Could you check a few things on this model? Use its own coordinates, in mm. Face numbers are marked on the shaded views. A direction names the side the tool comes from. Give positions to 0.01 mm unless a question says otherwise; leave off trailing zeros. Loops run counter-clockwise (first coordinate to the right, second up) from the corner with the lowest first, then second, coordinate; pieces in that order, holes last. Notation, with made-up numbers: (20.5, 55.25) - (24.5, 55.25) arc R10 cw to (24.5, 59.25) - close; hole circle Ø5 at (45.25, 34.25). An arc over 180 degrees is marked (long way). Answer in a Markdown table with one row per item. Add a question column.
```python
from build123d import *

# Parameters (mm, degrees)
SKETCH_1_W      = 3
SKETCH_1_H      = 17
EXTRUDE_1_DEPTH = 2.5
SKETCH_1_3_W    = 3
SKETCH_1_3_H    = 17
EXTRUDE_2_DEPTH = 2.5
FILLET_1_R      = 2


with BuildPart() as part:
    # Sketch 1 → Extrude 1 (new body)
    with BuildSketch(Plane(origin=(0, 0, 0), x_dir=(1, 0, 0), z_dir=(0, 1, 0))):
        Polygon((0, 15), (0, 17), (-15, 17), (-25, 6.390453713), (-25, 0), (0, 0), (0, 2), (-24.2, 2), (-24.2, 5), (0, 5), (0, 7), (-19.2, 7), (-19.2, 10), (0, 10), (0, 12), (-12.2, 12), (-12.2, 15), align=None)
        Polygon((5.5, 17), (0, 17), (0, 15), (-12.2, 15), (-12.2, 12), (0, 12), (0, 10), (-19.2, 10), (-19.2, 7), (0, 7), (0, 5), (-24.2, 5), (-24.2, 2), (0, 2), (0, 0), (5.5, 0), align=None)
        with Locations((7, 8.5)):
            Rectangle(SKETCH_1_W, SKETCH_1_H)
    extrude(amount=-EXTRUDE_1_DEPTH)

    # Sketch 1_3 → Extrude 2 (add)
    with BuildSketch(Plane(origin=(0, 0, 0), x_dir=(1, 0, 0), z_dir=(0, 1, 0))):
        Polygon((0, 15), (0, 17), (-15, 17), (-25, 6.390453713), (-25, 0), (0, 0), (0, 2), (-24.2, 2), (-24.2, 5), (0, 5), (0, 7), (-19.2, 7), (-19.2, 10), (0, 10), (0, 12), (-12.2, 12), (-12.2, 15), align=None)
        with Locations((7, 8.5)):
            Rectangle(SKETCH_1_3_W, SKETCH_1_3_H)
    extrude(amount=EXTRUDE_2_DEPTH)

    # Fillet 1
    fillet_1_edges = [part.edges().sort_by_distance(p)[0] for p in [
        (8.5, 0, -17),
        (8.5, 0, 0),
        (-25, 0, 0),
        (-25, 0, -6.390453713),
        (-15, 0, -17),
    ]]
    fillet(fillet_1_edges, radius=FILLET_1_R)


solid = part.part
```
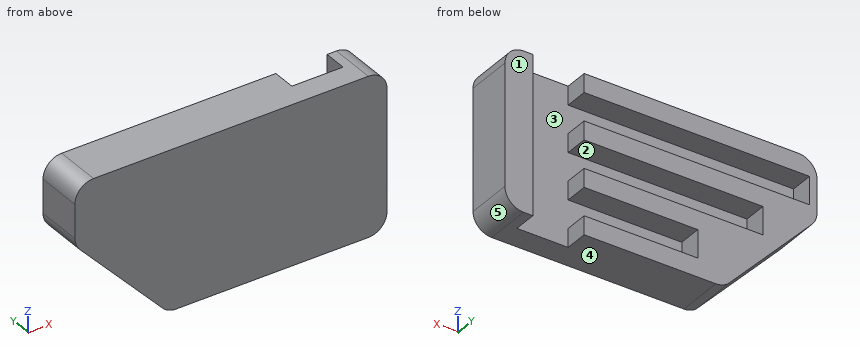
(1) We'd pull the mould along X, two halves only. Please class the marked faces 3, 4 and 5: pulls with the +X half, pulls with the -X half, needs draft (parallel to the pull), parting line crosses it, or undercut.
(2) I want a section at B-B on y = 1.2. Please give me the cut outline in (x, z).
(3) For pin 1 Ø0.6 at (y, z) = (0.5, -1.5) entering from +X; pin 2 Ø1.5 at (x, z) = (4, -2.5) entering from +Y; pin 3 Ø0.6 at (y, z) = (1.5, -16.5) entering from +X, each with a flat end and sliding along its axis, tell me the tip position at first contact or that it passes through.
(4) On a 3-axis mill with a long thin cutter (end or side, diameter ignored), from which of +Z, -Z, +X, -X, +Y, -Y can I reach the whole of each face in a straight line? I mean the marked faces 1 and 2. Say none if no direction works.
(5) Please list where these lines run through material, in increasing order: line 1 (X direction, y = 0.8, z = -4.5); line 2 (Z direction, x = -16.5, y = 2.15); line 3 (Z direction, x = -17.5, y = 2.3).
(6) I want a section at C-C on y = -1.35. Please give me the cut outline in (x, z).
(7) I want a section at A-A on x = -8.5. Please give me the cut outline in (y, z).
(8) I want a section at D-D on z = -3.25. Please give me the cut outline in (x, y).
Reported:
| question | item | result |
|---|---|---|
| 1 | face 3 | undercut |
| 1 | face 4 | needs draft |
| 1 | face 5 | pulls with the +X half |
| 2 | outline | (-25, -5.6) arc R2 ccw to (-24.46, -6.97) - (-15.59, -16.37) arc R2 ccw to (-14.14, -17) - (0, -17) - (0, -15) - (-12.2, -15) - (-12.2, -12) - (0, -12) - (0, -10) - (-19.2, -10) - (-19.2, -7) - (0, -7) - (0, -5) - (-24.2, -5) - (-24.2, -2) - (0, -2) - (0, 0) - (-23, 0) arc R2 ccw to (-25, -2) - close; (5.5, -17) - (6.5, -17) arc R2 ccw to (8.5, -15) - (8.5, -2) arc R2 ccw to (6.5, 0) - (5.5, 0) - close |
| 3 | pin 1 | x = 8.49 |
| 3 | pin 2 | y = 0 |
| 3 | pin 3 | x = 8.1 |
| 4 | face 1 | +Z, -Z, +X, -X, +Y |
| 4 | face 2 | +Y |
| 5 | line 1 | -25 to -24.2, 5.5 to 8.5 |
| 5 | line 2 | -15.41 to -10, -7 to -5, -2 to 0 |
| 5 | line 3 | -14.35 to -10, -7 to -5, -2 to 0 |
| 6 | outline | (-25, -5.6) arc R2 ccw to (-24.46, -6.97) - (-15.59, -16.37) arc R2 ccw to (-14.14, -17) - (6.5, -17) arc R2 ccw to (8.5, -15) - (8.5, -2) arc R2 ccw to (6.5, 0) - (-23, 0) arc R2 ccw to (-25, -2) - close |
| 7 | outline | (-2.5, -17) - (2.5, -17) - (2.5, -15) - (0, -15) - (0, -12) - (2.5, -12) - (2.5, -10) - (0, -10) - (0, -7) - (2.5, -7) - (2.5, -5) - (0, -5) - (0, -2) - (2.5, -2) - (2.5, 0) - (-2.5, 0) - close |
| 8 | outline | (-25, -2.5) - (8.5, -2.5) - (8.5, 2.5) - (5.5, 2.5) - (5.5, 0) - (-24.2, 0) - (-24.2, 2.5) - (-25, 2.5) - close |
